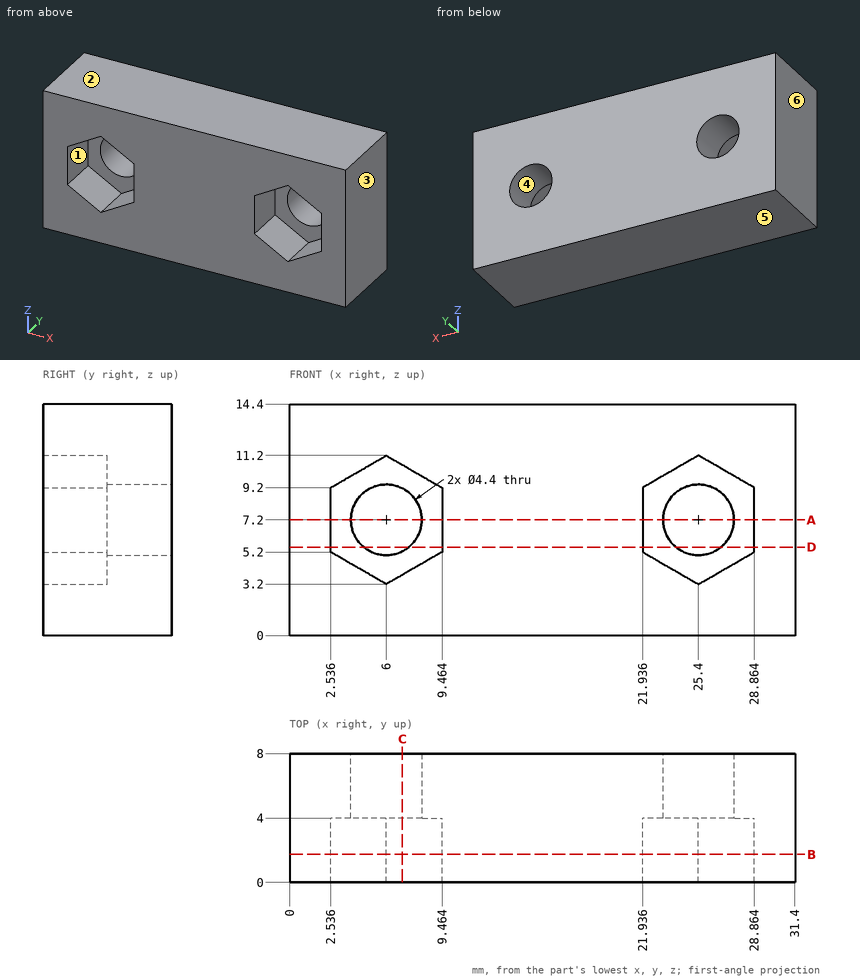
Job drawing, mm, ordinate dimensions from the low corner. One solid piece. A direction names the side the tool comes from. Coordinates: 2 decimals unless noted, no trailing zeros. Loops run counter-clockwise (first coordinate to the right, second up) from the corner with the lowest first, then second, coordinate; pieces in that order, holes last. Notation, with made-up numbers: (55, 50) - (83, 50) arc R13 cw to (83, 60) - close; hole circle Ø4 at (7, -36.5). An arc over 180 degrees is marked (long way). Write item = value, one per line. Start each with the question number.
Q1. Cut at A-A, the plane z = 7.2. List the corners of the cut face in (x, y), then the cut area to 3 significant figures.
Q2. Drill centre lines: L1, parallel to X at y = 6.6, z = 7.2; L2, parallel to X at y = 3.5, z = 4 (1 decimal); L3, parallel to Z at x = 25.4, y = 5.45. Where is each one in solid material? Low to high.
Q3. Cut at B-B, the plane y = 1.75. List the corners of the cut face in (x, z), then the cut area to 3 significant figures.
Q4. Cut at D-D, the plane z = 5.5. List the corners of the cut face in (x, y), then the cut area to 3 significant figures.
Q5. Which spindle directions (+Z, -Z, +X, -X, +Y, -Y) get a long thin tool onto all of the face, cutting with end or side? Do the marked faces 1 and 2. Say none if no direction does.
Q6. Pull direction X, two halves, no side cores. Call the marked faces 3, 4, 5 and 6: pulls with the +X half, pulls with the -X half, needs draft (parallel to the pull), parting line crosses it, or undercut.
Q7. Flat gauge pin, fed straight in: pin 1 Ø2 at (x, z) = (5.5, 9) entering from -Y. Where does the tip first touch, or does it go through?
Q8. Cut at C-C, the plane x = 7. List the corners of the cut face in (y, z).
Computed:
q1.outline = (0, 0) - (2.54, 0) - (2.54, 4) - (3.8, 4) - (3.8, 8) - (0, 8) - close; (8.2, 4) - (9.46, 4) - (9.46, 0) - (21.94, 0) - (21.94, 4) - (23.2, 4) - (23.2, 8) - (8.2, 8) - close; (27.6, 4) - (28.86, 4) - (28.86, 0) - (31.4, 0) - (31.4, 8) - (27.6, 8) - close
q1.area = 161 mm²
q2.L1 = 0 to 3.8, 8.2 to 23.2, 27.6 to 31.4
q2.L2 = 0 to 4.6, 7.4 to 24, 26.8 to 31.4
q2.L3 = 0 to 5, 9.4 to 14.4
q3.outline = (0, 0) - (31.4, 0) - (31.4, 14.4) - (0, 14.4) - close; hole (2.54, 5.2) - (6, 3.2) - (9.46, 5.2) - (9.46, 9.2) - (6, 11.2) - (2.54, 9.2) - close; hole (21.94, 5.2) - (25.4, 3.2) - (28.86, 5.2) - (28.86, 9.2) - (25.4, 11.2) - (21.94, 9.2) - close
q3.area = 369 mm²
q4.outline = (0, 0) - (2.54, 0) - (2.54, 4) - (4.6, 4) - (4.6, 8) - (0, 8) - close; (7.4, 4) - (9.46, 4) - (9.46, 0) - (21.94, 0) - (21.94, 4) - (24, 4) - (24, 8) - (7.4, 8) - close; (26.8, 4) - (28.86, 4) - (28.86, 0) - (31.4, 0) - (31.4, 8) - (26.8, 8) - close
q4.area = 173 mm²
q5.face_1 = -Y
q5.face_2 = +Z, +X, -X, +Y, -Y
q6.face_3 = pulls with the +X half
q6.face_4 = undercut
q6.face_5 = needs draft
q6.face_6 = pulls with the -X half
q7.pin_1 = 4
q8.outline = (0, 0) - (8, 0) - (8, 5.24) - (4, 5.24) - (4, 3.78) - (0, 3.78) - close; (0, 10.62) - (4, 10.62) - (4, 9.16) - (8, 9.16) - (8, 14.4) - (0, 14.4) - close
